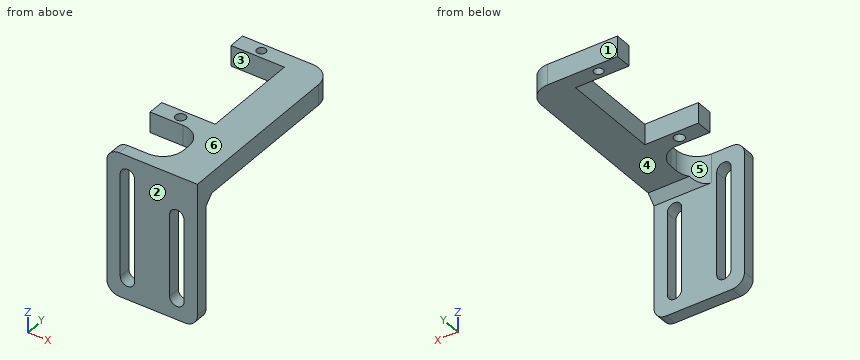
from build123d import *

# Parameters (mm, degrees)
SKETCH_1_W          = 12
SKETCH_1_H          = 4
SKETCH_1_R          = 1.1
SKETCH_1_R_2        = 1.25
EXTRUDE_1_DEPTH     = 2.5
EXTRUDE_START       = 2.5
SKETCH_1_5_W        = 22
SKETCH_1_5_H        = 3
EXTRUDE_3_DEPTH     = 35
SKETCH_2_R          = 1.75
CUT_EXTRUDE_1_DEPTH = 20
FILLET_1_R          = 5
FILLET_5_R          = 3
CHAMFER_1_SIZE      = 2
FILLET_6_R          = 5


with BuildPart() as part:
    # Sketch 1 → Extrude 1 (new, symmetric)
    # profile 1 of 3: a face of its own
    with BuildSketch(Plane.XY):
        Polygon((6, 16), (6, 12), (7, 12), (7, -12), (6, -12), (6, -16), (7, -16), (7, -28), (16, -28), (16, 16), align=None)
    # profile 2 of 3: a face of its own
    with BuildSketch(Plane.XY):
        with Locations((0, 14)):
            Rectangle(SKETCH_1_W, SKETCH_1_H)
        with Locations((0, 14)):
            Circle(SKETCH_1_R, mode=Mode.SUBTRACT)
    # profile 3 of 3: a face of its own
    with BuildSketch(Plane.XY):
        with Locations((0, -14)):
            Rectangle(SKETCH_1_W, SKETCH_1_H)
        with Locations((0, -14)):
            Circle(SKETCH_1_R_2, mode=Mode.SUBTRACT)
    extrude(amount=EXTRUDE_1_DEPTH, both=True)

    # Sketch 1_5 → Extrude 3 (add)
    with BuildSketch(Plane.XY.offset(EXTRUDE_START)):
        with Locations((5, -29.5)):
            Rectangle(SKETCH_1_5_W, SKETCH_1_5_H)
    extrude(amount=-EXTRUDE_3_DEPTH)

    # Sketch 2 → Cut-Extrude 1 (cut)
    with BuildSketch(Plane(origin=(0, -28, 0), x_dir=(1, 0, 0), z_dir=(0, 1, 0))):
        with BuildLine():
            ThreePointArc((0.75, 27.5), (-1, 25.75), (-2.75, 27.5))
            Line((-2.75, 27.5), (-2.75, 2.5))
            ThreePointArc((-2.75, 2.5), (-1, 4.25), (0.75, 2.5))
            Line((0.75, 2.5), (0.75, 27.5))
        make_face()
        with Locations((-1, 27.5)):
            Circle(SKETCH_2_R)
        with Locations((-1, 2.5)):
            Circle(SKETCH_2_R)
        with Locations((11, 7.5)):
            Circle(SKETCH_2_R)
        with BuildLine():
            ThreePointArc((12.75, 27.5), (11, 25.75), (9.25, 27.5))
            Line((9.25, 27.5), (9.25, 7.5))
            ThreePointArc((9.25, 7.5), (11, 9.25), (12.75, 7.5))
            Line((12.75, 7.5), (12.75, 27.5))
        make_face()
        with Locations((11, 27.5)):
            Circle(SKETCH_2_R)
    extrude(amount=-CUT_EXTRUDE_1_DEPTH, mode=Mode.SUBTRACT)

    # Fillet 1
    fillet_1_edges = [part.edges().sort_by_distance(p)[0] for p in [
        (7, -28, 0),
        (7, -16, 0),
    ]]
    fillet(fillet_1_edges, radius=FILLET_1_R)

    # Fillet 5
    fillet_5_edges = [part.edges().sort_by_distance(p)[0] for p in [
        (-6, -29.5, 2.5),
        (16, -29.5, -32.5),
        (-6, -29.5, -32.5),
    ]]
    fillet(fillet_5_edges, radius=FILLET_5_R)

    # Chamfer 1
    chamfer_1_edges = [part.edges().sort_by_distance(p)[0] for p in [
        (9, -28, -2.5),
    ]]
    chamfer(chamfer_1_edges, length=CHAMFER_1_SIZE)

    # Fillet 6
    fillet_6_edges = [part.edges().sort_by_distance(p)[0] for p in [
        (16, 16, 0),
    ]]
    fillet(fillet_6_edges, radius=FILLET_6_R)


solid = part.part
Verification items for the finished model (mm, model axes). Face numbers are marked on the shaded views. A direction names the side the tool comes from. Give positions to 0.01 mm unless a question says otherwise; leave off trailing zeros. Order: outer loops, then holes, each group sorted by start corner. A loop starts at its lowest first (then second) coordinate and runs counter-clockwise, first axis right, second up. Notation, with made-up numbers: M -5,15.25 L 4,15.25 A13 cw 4,24.25 Z; hole C -15.75,77.25 d6. An arc over 180 degrees is marked long. Use one line per item in the form item = value. Start each with the question number.
Q1. Section check D-D (y = -14). Enter the section's corners in (x, z).
Q2. Go/stop test with flat-tipped pins: pin 1 Ø0.6 at (y, z) = (-21.5, 1) entering from -X; pin 2 Ø1 at (x, y) = (9.5, 1.5) entering from -Z; pin 3 Ø10 at (x, z) = (1.5, -11) entering from +Y; pin 4 Ø12 at (x, y) = (-2, -1) entering from -Z. Record where each tip stops, or that it passes through.
Q3. Section check B-B (y = 14). Enter the section's corners in (x, z).
Q4. Section check A-A (z = -9.5). Enter the section's corners in (x, y).
Q5. Access from +Z, -Z, +X, -X, +Y, -Y to the whole of each face (thin tool, end or side, straight path). Record for the marked faces 4, 5 and 6.
Q6. Mould release check, pull along Y, two halves, no side actions. Record for the marked faces 1, 2 and 3: +Y half, -Y half, draft (parallel to the pull), parting line (faces both ways), or undercut.
Q7. Section check C-C (x = 0). Enter the section's corners in (y, z), then the cut area to 3 significant figures.
Q8. Scan lines: line 1 along Y through (x, z) = (0, 0.15); line 2 along Z through (x, y) = (7.5, -21.5); line 3 along Y through (x, z) = (10, -29). Record each from-to range of solid material in increasing order. Write a range as [from, to].
Evaluation:
q1.outline = M -6,-2.5 L -1.25,-2.5 L -1.25,2.5 L -6,2.5 Z; M 1.25,-2.5 L 16,-2.5 L 16,2.5 L 1.25,2.5 Z
q2.pin_1 = 7
q2.pin_2 = -2.5
q2.pin_3 = -28
q2.pin_4 = through
q3.outline = M -6,-2.5 L -1.1,-2.5 L -1.1,2.5 L -6,2.5 Z; M 1.1,-2.5 L 15,-2.5 L 15,2.5 L 1.1,2.5 Z
q4.outline = M -6,-31 L -2.75,-31 L -2.75,-28 L -6,-28 Z; M 0.75,-31 L 9.25,-31 L 9.25,-28 L 0.75,-28 Z; M 12.75,-31 L 16,-31 L 16,-28 L 12.75,-28 Z
q5.face_4 = -Z, +X, -X, +Y
q5.face_5 = +Z, -Z, -X
q5.face_6 = +Z, +X, -X, +Y, -Y
q6.face_1 = +Y half
q6.face_2 = -Y half
q6.face_3 = undercut
q7.outline = M -31,-32.5 L -28,-32.5 L -28,-28.94 L -31,-28.94 Z; M -31,-1.06 L -28,-1.06 L -28,2.5 L -31,2.5 Z; M -16,-2.5 L -15.25,-2.5 L -15.25,2.5 L -16,2.5 Z; M -12.75,-2.5 L -12,-2.5 L -12,2.5 L -12.75,2.5 Z; M 12,-2.5 L 12.9,-2.5 L 12.9,2.5 L 12,2.5 Z; M 15.1,-2.5 L 16,-2.5 L 16,2.5 L 15.1,2.5 Z
q7.area = 37.9 mm2
q8.line_1 = [-31, -28], [-16, -15.25], [-12.75, -12], [12, 12.9], [15.1, 16]
q8.line_2 = [-2.5, 2.5]
q8.line_3 = [-31, -28]
